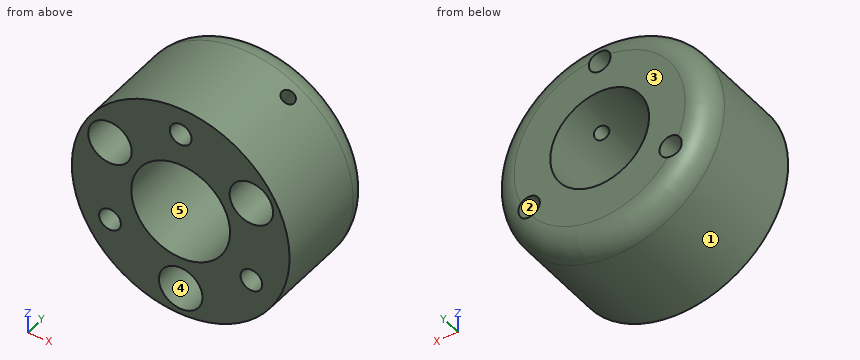
from build123d import *

# Parameters (mm, degrees)
SKETCH1_R               = 14
BOSS_EXTRUDE1_DEPTH     = 15
SKETCH2_R               = 1.4
SKETCH2_R_2             = 6.35
CUT_EXTRUDE1_DEPTH      = 25.839484697
BOSS_EXTRUDE2_DEPTH     = 2
CUT_EXTRUDE2_DEPTH      = 17
CUT_EXTRUDE2_DEPTH_BACK = 10
SKETCH4_R               = 0.9
SKETCH4_W               = 10.5
SKETCH4_H               = 2
SKETCH5_R               = 2.8
CUT_EXTRUDE3_DEPTH      = 5
FILLET1_R               = 3


with BuildPart() as part:
    # Sketch1 → Boss-Extrude1 (new body)
    with BuildSketch(Plane(origin=(0, 0, 0), x_dir=(1, 0, 0), z_dir=(0, 1, 0))):
        with Locations(Location((0, 0, 0), (0, 0, 270))):
            Circle(SKETCH1_R)
    extrude(amount=BOSS_EXTRUDE1_DEPTH)

    # Sketch2 → Cut-Extrude1 (cut, through all)
    with BuildSketch(Plane.XZ):
        with Locations(Location((0, 10.5, 0), (0, 0, 270))):
            Circle(SKETCH2_R)
        with Locations(Location((0, 0, 0), (0, 0, 270))):
            Circle(SKETCH2_R_2)
        with Locations(Location((9.09326674, -5.25, 0), (0, 0, 270))):
            Circle(SKETCH2_R)
        with Locations(Location((-9.09326674, -5.25, 0), (0, 0, 270))):
            Circle(SKETCH2_R)
    extrude(amount=-CUT_EXTRUDE1_DEPTH, mode=Mode.SUBTRACT)

    # Sketch3 → Boss-Extrude2 (add)
    with BuildSketch(Plane(origin=(0, 0, 0), x_dir=(1, 0, 0), z_dir=(0, 1, 0))):
        Polygon((0, 0), (9.09326674, -5.25), (0, -10.5), align=None)
    extrude(amount=-BOSS_EXTRUDE2_DEPTH)

    # Sketch4 → Cut-Extrude2 (cut, two sides: drawn at the far end of the back side and taken through both)
    with BuildSketch(Plane(origin=(4.54663337, 0, 7.875), x_dir=(0.8660254037844364, 0, -0.5000000000000041), z_dir=(0.500000000000004, 0, 0.8660254037844363)).offset(-CUT_EXTRUDE2_DEPTH_BACK)):
        with Locations(Location((0, 10, 0), (0, 0, 180))):
            Circle(SKETCH4_R)
        with Locations((0, -1)):
            Rectangle(SKETCH4_W, SKETCH4_H)
    extrude(amount=CUT_EXTRUDE2_DEPTH + CUT_EXTRUDE2_DEPTH_BACK, mode=Mode.SUBTRACT)

    # Sketch5 → Cut-Extrude3 (cut)
    with BuildSketch(Plane.XZ):
        with Locations(Location((9.09326674, 5.25, 0), (0, 0, 270))):
            Circle(SKETCH5_R)
        with Locations(Location((0, -10.5, 0), (0, 0, 270))):
            Circle(SKETCH5_R)
        with Locations(Location((-9.09326674, 5.25, 0), (0, 0, 270))):
            Circle(SKETCH5_R)
    extrude(amount=-CUT_EXTRUDE3_DEPTH, mode=Mode.SUBTRACT)

    # Fillet1
    # the kernel refuses this fillet: 3 mm, written as the material it takes off along each edge
    with BuildSketch(Plane(origin=(0, 15, 0), x_dir=(0, 0, 1), z_dir=(-1, 0, 0))) as fillet1_piece_1:
        with BuildLine():
            CenterArc((14 - FILLET1_R, -FILLET1_R), FILLET1_R, 0, 90)
            Line((14 - FILLET1_R, 0), (14, 0))
            Line((14, 0), (14, -FILLET1_R))
        make_face()
    revolve(axis=Axis((0, 15, 0), (0, 1, 0)), mode=Mode.SUBTRACT)


solid = part.part
Design review of the part built by this model. Coordinates are the model's own, in mm. Face numbers are marked on the shaded views. A direction names the side the tool comes from. Round coordinates to 2 decimals unless told otherwise and drop trailing zeros. Loops run counter-clockwise (first coordinate to the right, second up) from the corner with the lowest first, then second, coordinate; pieces in that order, holes last. Notation, with made-up numbers: M -30,-28 L -2,-28 A20 cw -2,4 Z; hole C 89,56 d9. An arc over 180 degrees is marked long. Answer as a JSON object with one key per item and string values.
Item 1: We need section D-D on y = 9.5. Give the boundary of the cut face in (x, z).
Answer sheet:
{"outline": "M 2.5,5.84 L 6.34,12.48 A14 ccw long 7.64,11.73 L 3.8,5.09 A6.35 cw long Z; hole C -9.09,-5.25 d2.8; hole C 0,10.5 d2.8; hole C 9.09,-5.25 d2.8"}
Item 2: Machinability: for the marked faces 4 and 5, which of the approach directions +Z, -Z, +X, -X, +Y, -Y give a long, thin tool a straight path to every point of the face, cutting with its end or side? Answer none if there is none.
Answer sheet:
{"face 4": "-Y", "face 5": "+Y, -Y"}
Item 3: We need section C-C on y = 12.75. Give the boundary of the cut face in (x, z), and give its area (3 significant figures).
Answer sheet:
{"outline": "C 0,0 d27.81; hole C -9.09,-5.25 d2.8; hole C 0,0 d12.7; hole C 0,10.5 d2.8; hole C 9.09,-5.25 d2.8", "area": "462 mm^2"}
Item 4: Clearance check with flat-ended pins moving along their axes: P1, Ø4, axis at x = 3.5, z = 1, coming from the +Y side; P2, Ø1.7, axis at x = -9.5, z = 4, coming from the -Y side; P3, Ø5, axis at x = -10, z = -11, coming from the +Y side; P4, Ø2, axis at x = 3.5, y = 9, coming from the +Z side (3 decimals). State where each tip first meets the part, or that it passes through.
Answer sheet:
{"P1": "passes through", "P2": "stops at y = 5", "P3": "stops at y = 14.67", "P4": "stops at z = 13.775"}
Item 5: The part is to be moulded in two halves that separate along X. For the marked faces 1, 2 and 3, say which applies: pulls with the +X half, pulls with the -X half, needs draft (parallel to the pull), parting line crosses it, or undercut.
Answer sheet:
{"face 1": "parting line crosses it", "face 2": "undercut", "face 3": "needs draft"}
Item 6: We need section A-A on z = 0. Give the boundary of the cut face in (x, y), and give its area (3 significant figures).
Answer sheet:
{"outline": "M -14,0 L -6.35,0 L -6.35,15 L -11,15 A3 ccw -14,12 Z; M 6.35,0 L 14,0 L 14,12 A3 ccw 11,15 L 6.35,15 Z", "area": "226 mm^2"}
Item 7: Wall thickness on L1, parallel to Z at x = 0, y = 6; L2, parallel to X at y = 3.5, z = 0; L3, parallel to Z at x = 2.5, y = 2: over which ranges is each line inside the solid? List them lowest first. Write a range as from..to.
Answer sheet:
{"L1": "z = -14..-6.35, 6.35..9.1, 11.9..14", "L2": "x = -14..-6.35, 6.35..14", "L3": "z = -13.77..-11.76, -9.24..-5.84, 5.84..13.77"}
Item 8: We need section B-B on x = 0. Give the boundary of the cut face in (y, z).
Answer sheet:
{"outline": "M 0,-14 L 12,-14 A3 ccw 15,-11 L 15,-6.35 L 0,-6.35 L 0,-7.7 L 5,-7.7 L 5,-13.3 L 0,-13.3 Z; M 0,6.35 L 15,6.35 L 15,9.1 L 0,9.1 Z; M 0,11.9 L 14.86,11.9 A3 ccw 12,14 L 0,14 Z"}
